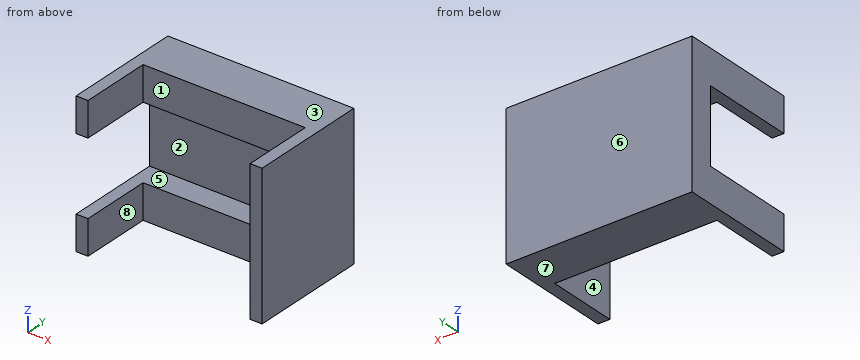
from build123d import *

# Parameters (mm, degrees)
SKETCH_1_W          = 5
SKETCH_1_H          = 30
EXTRUDE_1_DEPTH     = 60
SKETCH_2_W          = 68.186813186
SKETCH_2_H          = 31
CUT_EXTRUDE_1_DEPTH = 10
SKETCH_3_W          = 5
SKETCH_3_H          = 31
CUT_EXTRUDE_3_DEPTH = 40


with BuildPart() as part:
    # 草圖1 → 填料-伸長1 (new body)
    with BuildSketch(Plane.XY):
        Polygon((-56.41038016, 13.571428571), (-56.41038016, -6.428571429), (-51.41038016, -6.428571429), (16.776433026, -6.428571429), (21.776433026, -6.428571429), (21.776433026, 13.571428571), align=None)
        with Locations((-53.91038016, -21.428571429)):
            Rectangle(SKETCH_1_W, SKETCH_1_H)
        with Locations((19.276433026, -21.428571429)):
            Rectangle(SKETCH_1_W, SKETCH_1_H)
    extrude(amount=EXTRUDE_1_DEPTH)

    # 草圖2 → 除料-伸長1 (cut)
    with BuildSketch(Plane.XZ.offset(6.428571429)):
        with Locations((-17.316973567, 30)):
            Rectangle(SKETCH_2_W, SKETCH_2_H)
    extrude(amount=-CUT_EXTRUDE_1_DEPTH, mode=Mode.SUBTRACT)

    # 草圖3 → 除料-伸長3 (cut)
    with BuildSketch(Plane.XZ.offset(36.428571429)):
        with Locations((-53.91038016, 30)):
            Rectangle(SKETCH_3_W, SKETCH_3_H)
    extrude(amount=-CUT_EXTRUDE_3_DEPTH, mode=Mode.SUBTRACT)


solid = part.part
CAD build for the part. Positions are in the model's coordinates, mm. Face numbers are marked on the shaded views. A direction names the side the tool comes from. Give positions to 0.01 mm unless a question says otherwise; leave off trailing zeros. Write each loop counter-clockwise with the first axis right and the second up, starting at its lowest first coordinate (ties: lowest second). Pieces come first, ordered by that corner, then holes. Notation, with made-up numbers: (-39, 89) - (-20, 89) arc R9 cw to (-20, 98) - close; hole circle Ø5 at (14.25, -20.75). An arc over 180 degrees is marked (long way). Put each result on its own line as item: value.
(1) Saw through at A-A (y = -25). List the corners of the cut face in (x, z).
Working result:
outline: (-56.41, 0) - (-51.41, 0) - (-51.41, 14.5) - (-56.41, 14.5) - close; (-56.41, 45.5) - (-51.41, 45.5) - (-51.41, 60) - (-56.41, 60) - close; (16.78, 0) - (21.78, 0) - (21.78, 60) - (16.78, 60) - close
(2) Saw through at B-B (z = 54.5). List the corners of the cut face in (x, y).
Working result:
outline: (-56.41, -36.43) - (-51.41, -36.43) - (-51.41, -6.43) - (16.78, -6.43) - (16.78, -36.43) - (21.78, -36.43) - (21.78, 13.57) - (-56.41, 13.57) - close
(3) Pull direction Z, two halves, no side cores. Call the marked faces 1, 2 and 3: released by +Z, released by -Z, zero draft, split by the parting line, or undercut.
Working result:
face 1: zero draft
face 2: undercut
face 3: released by +Z
(4) Saw through at D-D (z = 30.5). List the corners of the cut face in (x, y), then the cut area to 3 significant figures.
Working result:
outline: (-56.41, 3.57) - (16.78, 3.57) - (16.78, -36.43) - (21.78, -36.43) - (21.78, 13.57) - (-56.41, 13.57) - close
area: 982 mm^2
(5) Wall check: L1, parallel to X at y = -21, z = 7.5; L2, parallel to Z at x = -53, y = -22; L3, parallel to Y at x = -33.5, z = 24.5. Give the ranges that are in metal, low to high.
Working result:
L1: -56.41 to -51.41, 16.78 to 21.78
L2: 0 to 14.5, 45.5 to 60
L3: 3.57 to 13.57
(6) Drop flat-ended pins along their axis: pin 1 Ø11.5 at (x, z) = (-6, 53) entering from -Y; pin 2 Ø8 at (x, z) = (-21.5, 23) entering from -Y; pin 3 Ø12 at (y, z) = (-22, 33.5) entering from -X; pin 4 Ø12 at (x, y) = (-32, -16) entering from +Z. Give the stop position or say it passes through.
Working result:
pin 1: y = -6.43
pin 2: y = 3.57
pin 3: x = 16.78
pin 4: through
(7) Saw through at C-C (x = -29). List the corners of the cut face in (y, z).
Working result:
outline: (-6.43, 0) - (13.57, 0) - (13.57, 60) - (-6.43, 60) - (-6.43, 45.5) - (3.57, 45.5) - (3.57, 14.5) - (-6.43, 14.5) - close
(8) Tool access for the marked faces 4, 5, 6, 7 and 8: list every direction of +Z, -Z, +X, -X, +Y, -Y with a clear straight run to the whole face (end or side of a thin tool).
Working result:
face 4: -Y
face 5: -X, -Y
face 6: +Z, -Z, +X, -X, +Y
face 7: -Z, +X, -X, +Y, -Y
face 8: +Z, -Z, -Y
